from build123d import *

# Parameters (mm, degrees)
SKETCH_R   = 53
SKETCH_R_2 = 3
PAD_DEPTH  = 5


with BuildPart() as part:
    # Sketch → Pad (new body)
    with BuildSketch(Plane.XY):
        Circle(SKETCH_R)
        Circle(SKETCH_R_2, mode=Mode.SUBTRACT)
    extrude(amount=PAD_DEPTH)

    # Sketch001 → Revolution (revolve)
    with BuildSketch(Plane.XZ):
        Polygon((53, 5), (47, 5), (47, 55), (48.75, 55), (48.75, 40), (51.25, 40), (51.25, 48), (53, 48), align=None)
    revolve(axis=Axis((0, 0, 0), (0, 0, 1)))


solid = part.part
Geometry check sheet. Reference: the model listing, model coordinates, mm. A direction names the side the tool comes from. Coordinates: 2 decimals unless noted, no trailing zeros. Order: outer loops, then holes, each group sorted by start corner. A loop starts at its lowest first (then second) coordinate and runs counter-clockwise, first axis right, second up. Notation, with made-up numbers: M 78,34 L 100,34 A11 cw 100,44 Z; hole C 17,72.25 d10. An arc over 180 degrees is marked long. Use CSV: the item, a comma, the result in double quotes.
Item 1: Cross-section at C-C on z = 13.5. Record the cut outline in (x, y).
Returned:
outline,"C 0,0 d106; hole C 0,0 d94"
Item 2: Mould release check, pull along X, two halves, no side actions. Record for faces 1 (the flat face through (11, 1, 0)), 2 (the flat face through (-1, -10, 5)), 3 (the cylindrical face through (28, 45, 24)): pulls with the +X half, pulls with the -X half, needs draft (parallel to the pull), parting line crosses it, or undercut.
Returned:
face 1,"needs draft"
face 2,"undercut"
face 3,"parting line crosses it"
Item 3: Thickness scan on line 1 along Y through (x, z) = (7.5, 46.5); line 2 along X through (y, z) = (-4.5, 42.5); line 3 along Y through (x, z) = (0, 27). Record the ranges inside material, lowest first.
Returned:
line 1,"y = -52.47 to -50.7, -48.17 to -46.4, 46.4 to 48.17, 50.7 to 52.47"
line 2,"x = -52.81 to -51.05, -48.54 to -46.78, 46.78 to 48.54, 51.05 to 52.81"
line 3,"y = -53 to -47, 47 to 53"
Item 4: Cross-section at D-D on x = -45. Record the cut outline in (y, z), then the cut area to 3 significant figures.
Returned:
outline,"M -28,0 L 28,0 L 28,48 L 24.53,48 L 24.53,40 L 18.75,40 L 18.75,55 L 13.56,55 L 13.56,5 L -13.56,5 L -13.56,55 L -18.75,55 L -18.75,40 L -24.53,40 L -24.53,48 L -28,48 Z"
area,"1,500 mm2"
Item 5: Gauge pin test, flat ends, axial feed: pin 1 Ø8 at (x, y) = (0, 0) entering from +Z; pin 2 Ø6 at (x, z) = (5.5, 45.5) entering from -Y; pin 3 Ø1.5 at (y, z) = (24, 32.5) entering from -X; pin 4 Ø10 at (y, z) = (2, 47) entering from -X. Record the tip position at first contact, or that the pin passes through.
Returned:
pin 1,"stops at z = 5"
pin 2,"stops at y = -52.94"
pin 3,"stops at x = -47.63"
pin 4,"stops at x = -53"
Item 6: Cross-section at A-A on y = 0. Record the cut outline in (x, z), then the cut area to 3 significant figures.
Returned:
outline,"M -53,0 L -3,0 L -3,5 L -47,5 L -47,55 L -48.75,55 L -48.75,40 L -51.25,40 L -51.25,48 L -53,48 Z; M 3,0 L 53,0 L 53,48 L 51.25,48 L 51.25,40 L 48.75,40 L 48.75,55 L 47,55 L 47,5 L 3,5 Z"
area,"1,000 mm2"
Item 7: Tool access check on faces 4 (the flat face through (26, 40, 55)), 5 (the cylindrical face through (-11.11, -50.03, 44.06)). Record the directions out of +Z, -Z, +X, -X, +Y, -Y that give a thin tool (end or side, any length) a straight path to the whole face; none if there is none.
Returned:
face 4,"+Z, +X, -X, +Y, -Y"
face 5,"+Z"
